```python
from build123d import *

# Parameters (mm, degrees)
BLANKSKE_W                  = 50
BLANKSKE_H                  = 9
BLANK_DEPTH                 = 12
TOOTHCUTSIM_DEPTH           = 53.201532545
TEETHCUTS_COUNT             = 17
TEETHCUTS_PITCH             = 3.14159265
SKETCH1_W                   = 50
SKETCH1_H                   = 10.518808777
CUT_EXTRUDE1_DEPTH          = 4
SKETCH2_W                   = 8
SKETCH2_H                   = 6.765098998
BOSS_EXTRUDE1_DEPTH         = 10
SKETCH3_W                   = 8
SKETCH3_H                   = 21
BOSS_EXTRUDE2_DEPTH         = 8
SKETCH4_W                   = 8
SKETCH4_H                   = 6
BOSS_EXTRUDE3_DEPTH         = 30
SKETCH5_W                   = 10
SKETCH5_H                   = 6
BOSS_EXTRUDE4_DEPTH         = 12
BODY_MOVE_COPY3_START       = -12
BODY_MOVE_COPY3_DEPTH       = 12
BODY_MOVE_COPY3_START_2     = 16
BODY_MOVE_COPY3_2_OUTLINE_W = 12
BODY_MOVE_COPY3_2_OUTLINE_H = 6
BODY_MOVE_COPY3_2_DEPTH     = 10
BODY_MOVE_COPY3_3_DEPTH     = 8
BODY_MOVE_COPY3_START_3     = 28
BODY_MOVE_COPY3_4_OUTLINE_W = 20
BODY_MOVE_COPY3_4_OUTLINE_H = 6
BODY_MOVE_COPY3_4_DEPTH     = 10
BODY_MOVE_COPY3_START_4     = 26
BODY_MOVE_COPY3_5_OUTLINE_W = 8
BODY_MOVE_COPY3_5_OUTLINE_H = 6
BODY_MOVE_COPY3_5_DEPTH     = 2
SKETCH8_R                   = 3
CUT_EXTRUDE2_DEPTH          = 4
FILLET1_R                   = 8
FILLET2_R                   = 13
SKETCH9_W                   = 8
SKETCH9_H                   = 20.359047751
BOSS_EXTRUDE5_DEPTH         = 6
FILLET3_R                   = 4
FILLET4_R                   = 12
CUT_EXTRUDE3_DEPTH          = 10
SKETCH11_W                  = 0.88887074
SKETCH11_H                  = 6.79103927
CUT_EXTRUDE4_DEPTH          = 10
CHAMFER10_SIZE              = 8


# Read off the part's stored shape, not the designer's step: Body-Move/Copy3
with BuildPart() as part:
    # BlankSke → Blank (new body)
    with BuildSketch(Plane.XY):
        with Locations((25, 4.5)):
            Rectangle(BLANKSKE_W, BLANKSKE_H)
    extrude(amount=-BLANK_DEPTH)

    # TooCutSkeSim → ToothCutSim (cut, through all)
    with BuildSketch(Plane.XY):
        Polygon((0.44443537, 6.75), (-0.44443537, 6.75), (-1.272613241, 9.0254), (1.272613241, 9.0254), align=None)
    toothcutsim = extrude(amount=-TOOTHCUTSIM_DEPTH, mode=Mode.SUBTRACT)

    # TeethCuts: ToothCutSim ×17
    with Locations(*[(i * TEETHCUTS_PITCH, 0, 0) for i in range(1, TEETHCUTS_COUNT)]):
        add(toothcutsim, mode=Mode.SUBTRACT)

    # Sketch1 → Cut-Extrude1 (cut)
    with BuildSketch(Plane.XY):
        with Locations((25, 5.259404389)):
            Rectangle(SKETCH1_W, SKETCH1_H)
    extrude(amount=-CUT_EXTRUDE1_DEPTH, mode=Mode.SUBTRACT)

    # Sketch2 → Boss-Extrude1 (add)
    with BuildSketch(Plane(origin=(50, 0, 0), x_dir=(0, 0, -1), z_dir=(1, 0, 0))):
        with Locations((8, 3.382549499)):
            Rectangle(SKETCH2_W, SKETCH2_H)
    extrude(amount=BOSS_EXTRUDE1_DEPTH)

    # Sketch3 → Boss-Extrude2 (add)
    with BuildSketch(Plane.XY.offset(-4)):
        with Locations((64, 10.5)):
            Rectangle(SKETCH3_W, SKETCH3_H)
    extrude(amount=-BOSS_EXTRUDE2_DEPTH)

    # Sketch4 → Boss-Extrude3 (add)
    with BuildSketch(Plane.XY.offset(-4)):
        with Locations((64, 18)):
            Rectangle(SKETCH4_W, SKETCH4_H)
    extrude(amount=BOSS_EXTRUDE3_DEPTH)

    # Sketch5 → Boss-Extrude4 (add)
    with BuildSketch(Plane.ZY.offset(-60)):
        with Locations((21, 18)):
            Rectangle(SKETCH5_W, SKETCH5_H)
    extrude(amount=BOSS_EXTRUDE4_DEPTH)

    # Body-Move/Copy3 outline → Body-Move/Copy3 (cut)
    with BuildSketch(Plane.XY.offset(BODY_MOVE_COPY3_START)):
        Polygon((68, 21), (60, 21), (60, 6.765098998), (50, 6.765098998), (50, 6.75), (49.82104703, 6.75), (49.002114003, 9), (48.387258147, 9), (47.56832512, 6.75), (46.67945438, 6.75), (45.860521353, 9), (45.245665497, 9), (44.42673247, 6.75), (43.53786173, 6.75), (42.718928703, 9), (42.104072847, 9), (41.28513982, 6.75), (40.39626908, 6.75), (39.577336053, 9), (38.962480197, 9), (38.14354717, 6.75), (37.25467643, 6.75), (36.435743403, 9), (35.820887547, 9), (35.00195452, 6.75), (34.11308378, 6.75), (33.294150753, 9), (32.679294897, 9), (31.86036187, 6.75), (30.97149113, 6.75), (30.152558103, 9), (29.537702247, 9), (28.71876922, 6.75), (27.82989848, 6.75), (27.010965453, 9), (26.396109597, 9), (25.57717657, 6.75), (24.68830583, 6.75), (23.869372803, 9), (23.254516947, 9), (22.43558392, 6.75), (21.54671318, 6.75), (20.727780153, 9), (20.112924297, 9), (19.29399127, 6.75), (18.40512053, 6.75), (17.586187503, 9), (16.971331647, 9), (16.15239862, 6.75), (15.26352788, 6.75), (14.444594853, 9), (13.829738997, 9), (13.01080597, 6.75), (12.12193523, 6.75), (11.303002203, 9), (10.688146347, 9), (9.86921332, 6.75), (8.98034258, 6.75), (8.161409553, 9), (7.546553697, 9), (6.72762067, 6.75), (5.83874993, 6.75), (5.019816903, 9), (4.404961047, 9), (3.58602802, 6.75), (2.69715728, 6.75), (1.878224253, 9), (1.263368397, 9), (0.44443537, 6.75), (0, 6.75), (0, 0), (68, 0), align=None)
    extrude(amount=BODY_MOVE_COPY3_DEPTH, mode=Mode.SUBTRACT)

    # Body-Move_Copy3 2 outline → Body-Move_Copy3 2 (cut)
    with BuildSketch(Plane.XY.offset(BODY_MOVE_COPY3_START_2)):
        with Locations((54, 18)):
            Rectangle(BODY_MOVE_COPY3_2_OUTLINE_W, BODY_MOVE_COPY3_2_OUTLINE_H)
    extrude(amount=BODY_MOVE_COPY3_2_DEPTH, mode=Mode.SUBTRACT)

    # Body-Move_Copy3 3 outline → Body-Move_Copy3 3 (add)
    with BuildSketch(Plane.XY):
        Polygon((68, 15), (60, 15), (60, 6.765098998), (50, 6.765098998), (50, 6.75), (49.82104703, 6.75), (49.002114003, 9), (48.387258147, 9), (47.56832512, 6.75), (46.67945438, 6.75), (45.860521353, 9), (45.245665497, 9), (44.42673247, 6.75), (43.53786173, 6.75), (42.718928703, 9), (42.104072847, 9), (41.28513982, 6.75), (40.39626908, 6.75), (39.577336053, 9), (38.962480197, 9), (38.14354717, 6.75), (37.25467643, 6.75), (36.435743403, 9), (35.820887547, 9), (35.00195452, 6.75), (34.11308378, 6.75), (33.294150753, 9), (32.679294897, 9), (31.86036187, 6.75), (30.97149113, 6.75), (30.152558103, 9), (29.537702247, 9), (28.71876922, 6.75), (27.82989848, 6.75), (27.010965453, 9), (26.396109597, 9), (25.57717657, 6.75), (24.68830583, 6.75), (23.869372803, 9), (23.254516947, 9), (22.43558392, 6.75), (21.54671318, 6.75), (20.727780153, 9), (20.112924297, 9), (19.29399127, 6.75), (18.40512053, 6.75), (17.586187503, 9), (16.971331647, 9), (16.15239862, 6.75), (15.26352788, 6.75), (14.444594853, 9), (13.829738997, 9), (13.01080597, 6.75), (12.12193523, 6.75), (11.303002203, 9), (10.688146347, 9), (9.86921332, 6.75), (8.98034258, 6.75), (8.161409553, 9), (7.546553697, 9), (6.72762067, 6.75), (5.83874993, 6.75), (5.019816903, 9), (4.404961047, 9), (3.58602802, 6.75), (2.69715728, 6.75), (1.878224253, 9), (1.263368397, 9), (0.44443537, 6.75), (0, 6.75), (0, 0), (68, 0), align=None)
    extrude(amount=BODY_MOVE_COPY3_3_DEPTH)



with BuildPart() as body_2:
    # Body-Move_Copy3 4 outline → Body-Move_Copy3 4 (new body)
    with BuildSketch(Plane.XY.offset(BODY_MOVE_COPY3_START_3)):
        with Locations((58, 18)):
            Rectangle(BODY_MOVE_COPY3_4_OUTLINE_W, BODY_MOVE_COPY3_4_OUTLINE_H)
    extrude(amount=BODY_MOVE_COPY3_4_DEPTH)


with BuildPart() as part_1:
    add(part.part)

    add(body_2.part)  # Body-Move_Copy3 5 merges body 2
    # Body-Move_Copy3 5 outline → Body-Move_Copy3 5 (add)
    with BuildSketch(Plane.XY.offset(BODY_MOVE_COPY3_START_4)):
        with Locations((64, 18)):
            Rectangle(BODY_MOVE_COPY3_5_OUTLINE_W, BODY_MOVE_COPY3_5_OUTLINE_H)
    extrude(amount=BODY_MOVE_COPY3_5_DEPTH)

    # Sketch8 → Cut-Extrude2 (cut)
    with BuildSketch(Plane.XZ):
        with Locations(Location((48, 4, 0), (0, 0, 270))):
            Circle(SKETCH8_R)
    extrude(amount=-CUT_EXTRUDE2_DEPTH, mode=Mode.SUBTRACT)

    # Fillet1
    fillet1_edges = [part_1.edges().sort_by_distance(p)[0] for p in [
        (60, 6.765098998, 4),
    ]]
    fillet(fillet1_edges, radius=FILLET1_R)

    # Fillet2
    fillet2_edges = [part_1.edges().sort_by_distance(p)[0] for p in [
        (68, 0, 4),
    ]]
    fillet(fillet2_edges, radius=FILLET2_R)

    # Sketch9 → Boss-Extrude5 (add)
    with BuildSketch(Plane(origin=(0, 21, 0), x_dir=(1, 0, 0), z_dir=(0, 1, 0))):
        with Locations((52, -48.179523876)):
            Rectangle(SKETCH9_W, SKETCH9_H)
    extrude(amount=-BOSS_EXTRUDE5_DEPTH)

    # Fillet3
    fillet3_edges = [part_1.edges().sort_by_distance(p)[0] for p in [
        (60, 18, 28),
        (56, 18, 38),
    ]]
    fillet(fillet3_edges, radius=FILLET3_R)

    # Fillet4
    fillet4_edges = [part_1.edges().sort_by_distance(p)[0] for p in [
        (48, 18, 28),
        (68, 18, 38),
    ]]
    fillet(fillet4_edges, radius=FILLET4_R)

    # Sketch10 → Cut-Extrude3 (cut)
    with BuildSketch(Plane(origin=(0, 0, 0), x_dir=(-1, 0, 0), z_dir=(0, 0, -1))):
        Polygon((-18.40512053, 6.75), (-18.40512053, 0), (5.217531279, 0), (5.217531279, 6.75), (5.217531279, 11.737070905), (-18.40512053, 11.737070905), align=None)
    extrude(amount=-CUT_EXTRUDE3_DEPTH, mode=Mode.SUBTRACT)

    # Sketch11 → Cut-Extrude4 (cut)
    with BuildSketch(Plane(origin=(0, 0, 0), x_dir=(-1, 0, 0), z_dir=(0, 0, -1))):
        with Locations((-18.8495559, 3.354480365)):
            Rectangle(SKETCH11_W, SKETCH11_H)
    extrude(amount=-CUT_EXTRUDE4_DEPTH, mode=Mode.SUBTRACT)

    # Chamfer10
    chamfer10_edges = [part_1.edges().sort_by_distance(p)[0] for p in [
        (56, 18, 58.359047751),
    ]]
    chamfer(chamfer10_edges, length=CHAMFER10_SIZE - 0.0001)  # a hair under: the kernel refuses the full size


solid = part_1.part
```
Model file for the job. Use its own axes, mm. A direction names the side the tool comes from. Coordinates: 2 decimals unless noted, no trailing zeros. Order: outer loops, then holes, each group sorted by start corner. A loop starts at its lowest first (then second) coordinate and runs counter-clockwise, first axis right, second up. Notation, with made-up numbers: (32.5, 54.25) -> (59.5, 54.25) arc R13 cw to (59.5, 63.25) -> close; hole circle Ø9 at (19, 10). An arc over 180 degrees is marked (long way). Return JSON: item names as keys, results as strings.
Item 1: Slice it at C-C (z = 53). Write the cut outline in (x, y).
Model answer:
{"outline": "(48, 15) -> (53.36, 15) -> (53.36, 21) -> (48, 21) -> close"}
Item 2: 3-axis set-ups, long thin cutter, end or side, ignore diameter. For faces 1 (the face through (51, 2, 4)), 2 (the face through (64.293, 3.909, 4.056)), 3 (the face through (46.276, 7.859, 3.944)): which of +Z, -Z, +X, -X, +Y, -Y reach the whole face in a straight line?
Model answer:
{"face 1": "-Y", "face 2": "+Z, -Z, +X, -Y", "face 3": "+Z, -Z, +Y"}
Item 3: Mould opens along X. For faces 4 (the face through (49.417, 7.859, 3.944)), 5 (the face through (56, 18, 46)), 6 (the face through (19.71, 7.89, 3.94)), 7 (the face through (58, 21, 29)) say: pulls with the +X half, pulls with the -X half, needs draft (parallel to the pull), parting line crosses it, or undercut.
Model answer:
{"face 4": "undercut", "face 5": "pulls with the +X half", "face 6": "pulls with the -X half", "face 7": "needs draft"}
Item 4: Pin check, flat tips, straight feed: P1, Ø0.6, axis at x = 50.5, z = 4, coming from the +Y side; P2, Ø3, axis at y = 17, z = 50.5, coming from the -X side; P3, Ø7.5, axis at x = 44.5, y = 5.5, coming from the +Z side; P4, Ø10, axis at x = 39.5, y = 14.5, coming from the +Z side. Stop position of each tip, or through.
Model answer:
{"P1": "stops at y = 6.77", "P2": "stops at x = 48", "P3": "stops at z = 8", "P4": "passes through"}
Item 5: Wall check: line 1 along Z through (x, y) = (22, 6); line 2 along X through (y, z) = (1.25, 4); line 3 along Y through (x, z) = (66, 26.5). Give the ranges that are in metal, low to high. Write a range as from..to.
Model answer:
{"line 1": "z = 0..8", "line 2": "x = 19.29..45, 51..60.56", "line 3": "y = 15..21"}
Item 6: Slice it at A-A (y = 2.75). Write the cut outline in (x, z).
Model answer:
{"outline": "(19.29, 0) -> (63, 0) -> (63, 8) -> (19.29, 8) -> close; hole circle Ø6 at (48, 4)"}
Item 7: Slice it at B-B (z = 19.5). Write the cut outline in (x, y), then the cut area to 3 significant figures.
Model answer:
{"outline": "(60, 15) -> (68, 15) -> (68, 21) -> (60, 21) -> close", "area": "48.0 mm²"}
